Autodesk Inventor part; units mm, degrees
ref_plane "YZ Plane" through (0, 0, 0) normal (1, 0, 0) x (0, 1, 0)
ref_plane "XZ Plane" through (0, 0, 0) normal (0, 1, 0) x (-1, 0, 0)
ref_plane "XY Plane" through (0, 0, 0) normal (0, 0, 1) x (1, 0, 0)
sketch "Esboço1" plane through (0, 0, 0) normal (0, 1, 0) x (-1, 0, 0)
  line L0 (0, 0) -> (40, 0)
  line L1 (40, 0) -> (40, -40)
  line L2 (40, -40) -> (0, -40)
  line L3 (0, -40) -> (0, 0)
  line L4 (0, 0) -> (1.5, 0)
  line L5 (1.5283, -1.4997) -> (38.5283, -1.4997)
  line L6 (38.5283, -1.4997) -> (38.5283, -38.4997)
  line L7 (38.5283, -38.4997) -> (1.5283, -38.4997)
  line L8 (1.5283, -38.4997) -> (1.5283, -1.4997)
  line L9 (1804, 0) -> (1764, 0)
  line L10 (1764, 0) -> (1764, -40)
  line L11 (1764, -40) -> (1804, -40)
  line L12 (1804, -40) -> (1804, 0)
  line L13 (1804, 0) -> (1802.5, 0)
  line L14 (1804, -1.4997) -> (1804, 0)
  line L15 (1802.5, -1.4997) -> (1765.5, -1.4997)
  line L16 (1765.5, -1.4997) -> (1765.5, -38.4997)
  line L17 (1765.5, -38.4997) -> (1802.5, -38.4997)
  line L18 (1802.5, -38.4997) -> (1802.5, -1.4997)
  line L19 (38.5283, -1.4997) -> (1.5283, -1.4997)
  line L20 (1.5283, -1.4997) -> (1.5283, -38.4997)
  line L21 (1.5283, -38.4997) -> (38.5283, -38.4997)
  line L22 (38.5283, -38.4997) -> (38.5283, -1.4997)
  dimension "d0" = 40
  dimension "d1" = 40
  dimension "d2" = 1.5
  dimension "d3" = 1.5
  dimension "d4" = 37
  dimension "d5" = 37
  dimension "d6" = 1804
  dimension "d8" = 40
  dimension "d9" = 40
  dimension "d10" = 1.5
  dimension "d11" = 37
  dimension "d12" = 37
  dimension "d15" = 37
  dimension "d16" = 37
extrude "Extrusão1" add sketch "Esboço1" along normal blind 400
sketch "Esboço2" plane through (0, 0, 0) normal (0, 1, 0) x (-1, 0, 0)
  line L0 (38.4659, -1.6068) -> (1.4659, -1.6068)
  line L1 (1.4659, -1.6068) -> (1.4659, -38.6068)
  line L2 (1.4659, -38.6068) -> (38.4659, -38.6068)
  line L3 (38.4659, -38.6068) -> (38.4659, -1.6068)
  point P0 (0, 0)
  dimension "d17" = 37
  dimension "d18" = 37
extrude "Extrusão2" add sketch "Esboço2" along normal blind 1.5
sketch "Esboço3" plane through (0, 0, 0) normal (0, 1, 0) x (-1, 0, 0)
  line L0 (1802.5, -38.4997) -> (1765.5, -38.4997)
  line L1 (1765.5, -38.4997) -> (1765.5, -1.4997)
  line L2 (1802.5, -38.4997) -> (1765.5, -38.4997)
  line L3 (1765.5, -38.4997) -> (1765.5, -1.4997)
  line L4 (1765.5, -1.4997) -> (1802.5, -1.4997)
  line L5 (1802.5, -1.4997) -> (1802.5, -38.4997)
  point P0 (0, 0)
extrude "Extrusão3" add sketch "Esboço3" along normal blind 1.5
sketch "Esboço4" plane through (0, 0, 0) normal (0, 0, 1) x (1, 0, 0)
  line L0 (-40, 0) -> (-40, 400)
  line L1 (-40, 0) -> (-1764, 0)
  line L2 (-1764, 0) -> (-1764, 44.8822)
  line L3 (-40, 44.8822) -> (-40, 0)
  line L4 (-1764, 0) -> (-40, 0)
  line L5 (-40, 0) -> (-40, 40)
  line L6 (-40, 40) -> (-1764, 40)
  line L7 (-1764, 40) -> (-1764, 0)
  point P0 (0, 0)
  dimension "d23" = 1724
  dimension "d24" = 1724
  dimension "d25" = 40
sketch "Esboço7" plane through (0, 0, 0) normal (1, 0, 0) x (0, 1, 0)
  line L0 (0, 0) -> (1.5, 0)
  line L1 (1.5, 0) -> (1.5, -1.5)
  line L2 (1.5, -1.5) -> (0, -1.5)
  line L3 (0, -1.5) -> (0, 0)
  line L4 (1.5, -1.4997) -> (400, -1.4997)
  line L5 (1.5, -1.4997) -> (38.5, -1.4997)
  line L6 (38.5, -1.4997) -> (38.5, -38.4997)
  line L7 (38.5, -38.4997) -> (1.5, -38.4997)
  line L8 (1.5, -38.4997) -> (1.5, -1.4997)
  line L9 (0, 0) -> (400, 0)
  line L10 (0, 0) -> (40, 0)
  line L11 (40, 0) -> (40, -40)
  line L12 (40, -40) -> (0, -40)
  line L13 (0, -40) -> (0, 0)
  dimension "d44" = 1.5
  dimension "d45" = 1.5
  dimension "d46" = 37
  dimension "d47" = 37
  dimension "d48" = 40
  dimension "d49" = 40
extrude "Extrusão6" add sketch "Esboço7" against normal blind 1804 contours L0 L1 L2 L3 | L9 L11 L4 L1 | L2 L8 L7 L6 L4 L11 L12 L13
sketch "Esboço9" plane through (0, 0, -40) normal (0, 0, -1) x (-1, 0, 0)
  line L0 (40, 40) -> (1764, 40)
  line L1 (0, 0) -> (0, 400)
  point P0 (842, 20)
  point P1 (962, 20)
  point P2 (0, 373)
  dimension "d87" = 20
  dimension "d88" = 20
  dimension "d89" = 120
  dimension "d90" = 842
hole "Furo2" at (-842, 20, -40) at (-962, 20, -40) direction (0, 0, 1) diameter 10 depth 200
sketch "Esboço10" plane through (-1764, 40, -40) normal (0, 1, 0) x (1, 0, 0)
  line L0 (1764, -40) -> (1764, 0)
  line L1 (1724, -40) -> (0, -40)
  point P0 (862, -20)
  dimension "d98" = 902
  dimension "d99" = 20
hole "Furo3" at (-902, 40, -20) direction (0, -1, 0) diameter 10 depth 200
chamfer "Chanfro8" distance 30 angle 45 1 edges at (0, 400, -20)
chamfer "Chanfro9" distance 10 angle 45 1 edges at (-40, 400, -20)
chamfer "Chanfro10" distance 10 angle 45 1 edges at (-1764, 400, -20)
chamfer "Chanfro11" distance 30 angle 45 1 edges at (-1804, 400, -20)
properties part number "Base_Fundo_Suporte_Lamina"
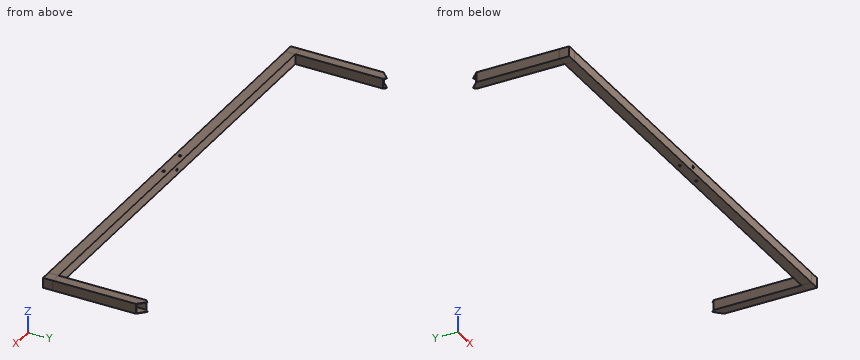
Geometry check sheet. Reference: the model listing, model coordinates, mm. Give positions to 0.01 mm unless a question says otherwise; leave off trailing zeros. Write each loop counter-clockwise with the first axis right and the second up, starting at its lowest first coordinate (ties: lowest second). Pieces come first, ordered by that corner, then holes.
1) Thickness scan on line 1 (X direction, y = 258, z = -18.5); line 2 (X direction, y = 20, z = -39); line 3 (Y direction, x = -281.5, z = -8). Record the ranges inside material, lowest first.
Values follow:
line 1: x = -1804 to -1802.5, -1765.5 to -1764, -40 to -38.53, -1.53 to 0
line 2: x = -1804 to -967, -957 to -847, -837 to 0
line 3: y = 0 to 1.5, 38.5 to 40
2) Cross-section at C-C (x = -218.5). Record the boundary of the cut face in (y, z).
Values follow:
outline: (0, -40) - (40, -40) - (40, 0) - (0, 0) - close; hole (1.5, -38.5) - (38.5, -38.5) - (38.5, -1.5) - (1.5, -1.5) - close
3) Cross-section at A-A (y = 70.5). Record the boundary of the cut face in (x, z), plus the area to 3 significant figures.
Values follow:
outline: (-1804, -40) - (-1764, -40) - (-1764, 0) - (-1804, 0) - close; (-40, -40) - (0, -40) - (0, 0) - (-40, 0) - close; hole (-1802.5, -38.5) - (-1765.5, -38.5) - (-1765.5, -1.5) - (-1802.5, -1.5) - close; hole (-38.53, -38.5) - (-1.53, -38.5) - (-1.53, -1.5) - (-38.53, -1.5) - close
area: 462 mm2
4) Cross-section at B-B (z = -31). Record the boundary of the cut face in (x, y), plus the area to 3 significant figures.
Values follow:
outline: (-1804, 0) - (0, 0) - (0, 370) - (-1.53, 371.53) - (-1.53, 40) - (-38.53, 40) - (-38.53, 391.47) - (-40, 390) - (-40, 40) - (-1764, 40) - (-1764, 390) - (-1765.5, 391.5) - (-1765.5, 40) - (-1802.5, 40) - (-1802.5, 371.5) - (-1804, 370) - close; hole (-1802.5, 1.5) - (-1765.5, 1.5) - (-1765.5, 38.5) - (-1802.5, 38.5) - close; hole (-1764, 1.5) - (-40, 1.5) - (-40, 38.5) - (-1764, 38.5) - close; hole (-38.53, 1.5) - (-1.53, 1.5) - (-1.53, 38.5) - (-38.53, 38.5) - close
area: 7,680 mm2
5) Go/stop test with flat-tipped pins: pin 1 Ø5 at (x, z) = (-573.5, -10) entering from -Y; pin 2 Ø8 at (x, z) = (-1434.5, -25.5) entering from +Y; pin 3 Ø8 at (x, y) = (-842, 20) entering from -Z. Record where each tip stops, or that it passes through.
Values follow:
pin 1: stops at y = 0
pin 2: stops at y = 40
pin 3: passes through
